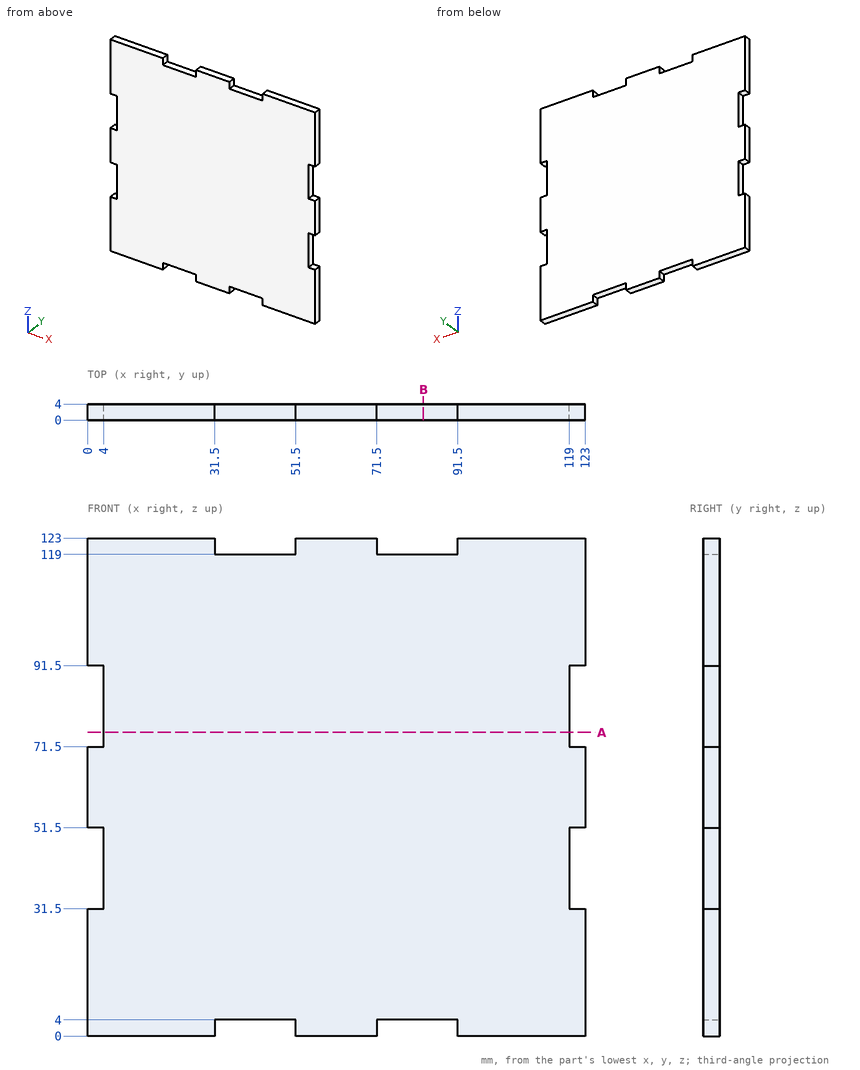
Can you work these out from the drawing? Everything is in mm from the part's minimum corner. Give positions to 0.01 mm unless a question says otherwise; leave off trailing zeros. Order: outer loops, then holes, each group sorted by start corner. A loop starts at its lowest first (then second) coordinate and runs counter-clockwise, first axis right, second up.
Item 1: If we section it at A-A, the plane z = 75: Write out the boundary of the cut face in (x, y), plus the area to 3 significant figures.
Item 2: If we section it at B-B, the plane x = 83: Write out the boundary of the cut face in (y, z), plus the area to 3 significant figures.
Item 3: I'm going to push flat-ended pins straight in: pin 1 (2 mm diameter, centred on y = 3, z = 47, fed in from +X); pin 2 (1 mm diameter, centred on x = 107.5, y = 3.5, fed in from -Z); pin 3 (1.2 mm diameter, centred on y = 1.5, z = 84.5, fed in from -X). Where does each tip first touch, or does it pass through?
Item 4: I need wall thicknesses on line 1 (Z direction, x = 42.5, y = 1.8). Which ranges of the line are inside material? Lowest first, please.
Values:
1. outline: (4, 0) - (119, 0) - (119, 4) - (4, 4) - close
1. area: 460 mm2
2. outline: (0, 4) - (4, 4) - (4, 119) - (0, 119) - close
2. area: 460 mm2
3. pin 1: stops at x = 119
3. pin 2: stops at z = 0
3. pin 3: stops at x = 4
4. line 1: z = 4 to 119
